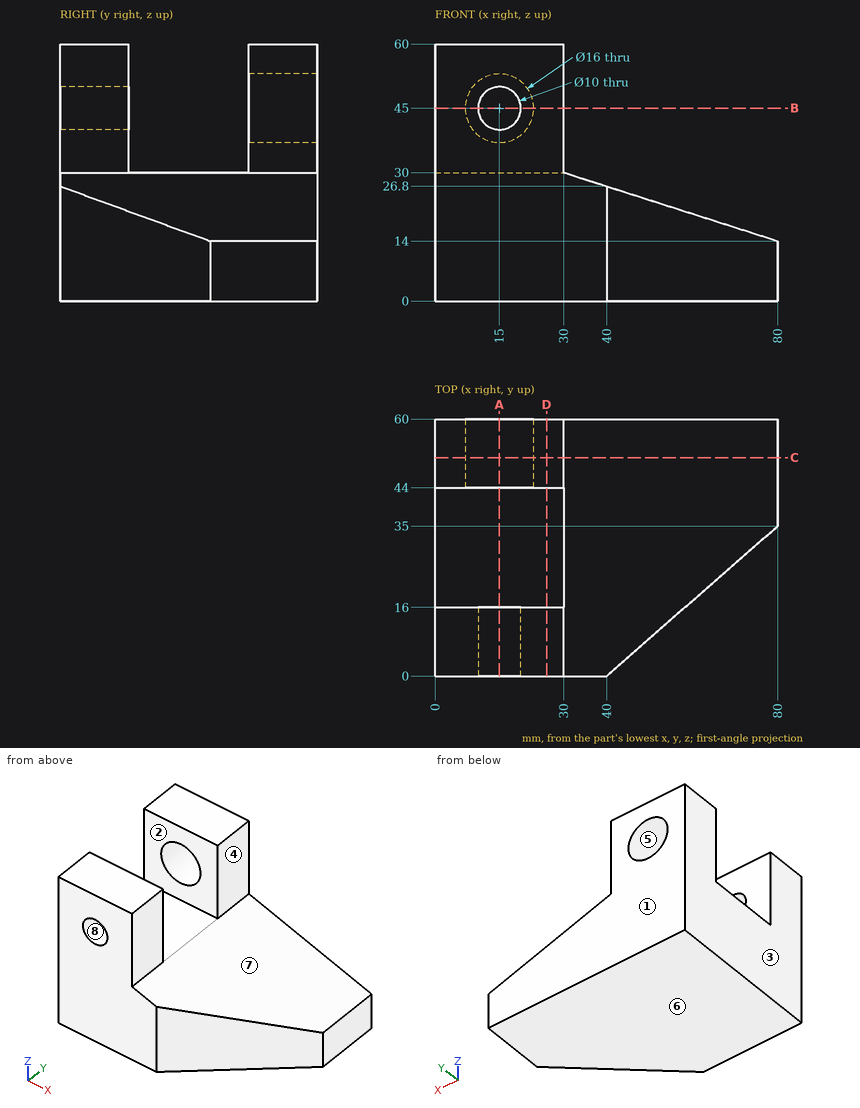
Here's the drawing with two shaded views (mm, measured from the low corner). I have some questions. A direction names the side the tool comes from. Coordinates: 2 decimals unless noted, no trailing zeros. Order: outer loops, then holes, each group sorted by start corner. A loop starts at its lowest first (then second) coordinate and runs counter-clockwise, first axis right, second up. Notation, with made-up numbers: (0.25, -3.75) - (57.25, -3.75) arc R24 cw to (57.25, 15.25) - close; hole circle Ø2 at (-7, 28.5). An arc over 180 degrees is marked (long way). Answer in a Markdown table with one row per item. Add a question column.
(1) If we section it at C-C, the plane y = 51: Please give me the cut outline in (x, z), then the cut area to 3 significant figures.
(2) If we section it at B-B, the plane z = 45: Please give me the cut outline in (x, y), then the cut area to 3 significant figures.
(3) If we section it at D-D, the plane x = 26: Please give me the cut outline in (y, z), then the cut area to 3 significant figures.
(4) On a 3-axis mill with a long thin cutter (end or side, diameter ignored), from which of +Z, -Z, +X, -X, +Y, -Y can I reach the whole of each face in a straight line? I mean the marked faces 1, 2, 3, 4 and 5. Say none if no direction works.
(5) If we section it at A-A, the plane x = 15: Please give me the cut outline in (y, z).
(6) If we mould it in two halves opening along X, with no side actions, what happens to the marked faces 6, 7 and 8? For each: released by +X, released by -X, zero draft, split by the parting line, or undercut.
(7) Will these pins go through, and if not, where does the flat tip stop? pin 1 (14 mm diameter, centred on x = 13.5, y = 25.5, fed in from +Z); pin 2 (13 mm diameter, centred on y = 52, z = 37.5, fed in from +X); pin 3 (6 mm diameter, centred on x = 55, y = 13.5, fed in from +Z).
(8) I need wall thicknesses on L1, parallel to Z at x = 15, y = 48; L2, parallel to X at y = 44.5, z = 31. Which ranges of each line are inside material? Lowest first, please.
Results are:
| question | item | result |
|---|---|---|
| 1 | outline | (0, 0) - (80, 0) - (80, 14) - (30, 30) - (30, 60) - (0, 60) - close; hole circle Ø16 at (15, 45) |
| 1 | area | 2,700 mm2 |
| 2 | outline | (0, 0) - (10, 0) - (10, 16) - (0, 16) - close; (0, 44) - (7, 44) - (7, 60) - (0, 60) - close; (20, 0) - (30, 0) - (30, 16) - (20, 16) - close; (23, 44) - (30, 44) - (30, 60) - (23, 60) - close |
| 2 | area | 544 mm2 |
| 3 | outline | (0, 0) - (60, 0) - (60, 60) - (44, 60) - (44, 30) - (16, 30) - (16, 60) - (0, 60) - close |
| 3 | area | 2,760 mm2 |
| 4 | face 1 | +Z, -Z, +X, -X, +Y |
| 4 | face 2 | +Z, +X, -X |
| 4 | face 3 | +Z, -Z, -X, +Y, -Y |
| 4 | face 4 | +Z, +X, +Y, -Y |
| 4 | face 5 | +Y |
| 5 | outline | (0, 0) - (60, 0) - (60, 37) - (44, 37) - (44, 30) - (16, 30) - (16, 40) - (0, 40) - close; (0, 50) - (16, 50) - (16, 60) - (0, 60) - close; (44, 53) - (60, 53) - (60, 60) - (44, 60) - close |
| 6 | face 6 | zero draft |
| 6 | face 7 | released by +X |
| 6 | face 8 | undercut |
| 7 | pin 1 | stops at z = 30 |
| 7 | pin 2 | stops at x = 30 |
| 7 | pin 3 | stops at z = 22.96 |
| 8 | L1 | z = 0 to 37, 53 to 60 |
| 8 | L2 | x = 0 to 30 |
